from build123d import *

# Parameters (mm, degrees)
SKETCH1_W           = 10.16
SKETCH1_H           = 5.08
BOSS_EXTRUDE1_DEPTH = 63.5
SKETCH2_W           = 2.1082
SKETCH2_H           = 6.073980388
CUT_EXTRUDE1_DEPTH  = 6
SKETCH3_W           = 0.5
SKETCH3_H           = 2.1082
CUT_EXTRUDE2_DEPTH  = 6
SKETCH4_W           = 6.35
SKETCH4_H           = 6.35
BOSS_EXTRUDE2_DEPTH = 60
FILLET3_R           = 4
FILLET4_R           = 0.5
FILLET6_R           = 5
FILLET10_R          = 5


with BuildPart() as part:
    # Sketch1 → Boss-Extrude1 (new body)
    with BuildSketch(Plane(origin=(0, 0, 0), x_dir=(0, 0, -1), z_dir=(1, 0, 0))):
        with Locations((5.08, 2.54)):
            Rectangle(SKETCH1_W, SKETCH1_H)
    extrude(amount=BOSS_EXTRUDE1_DEPTH)

    # Sketch2 → Cut-Extrude1 (cut)
    with BuildSketch(Plane(origin=(0, 5.08, 0), x_dir=(1, 0, 0), z_dir=(0, 1, 0))):
        with Locations((6.1341, 7.123009806)):
            Rectangle(SKETCH2_W, SKETCH2_H)
    extrude(amount=-CUT_EXTRUDE1_DEPTH, mode=Mode.SUBTRACT)

    # Sketch3 → Cut-Extrude2 (cut)
    with BuildSketch(Plane(origin=(0, 5.08, 0), x_dir=(1, 0, 0), z_dir=(0, 1, 0))):
        with Locations((4.83, 5.140119612)):
            Rectangle(SKETCH3_W, SKETCH3_H)
    extrude(amount=-CUT_EXTRUDE2_DEPTH, mode=Mode.SUBTRACT)

    # Sketch4 → Boss-Extrude2 (add)
    with BuildSketch(Plane(origin=(63.5, 0, 0), x_dir=(0, 0, -1), z_dir=(1, 0, 0))):
        with Locations((3.175, 3.175)):
            Rectangle(SKETCH4_W, SKETCH4_H)
    extrude(amount=BOSS_EXTRUDE2_DEPTH)

    # Fillet3
    # the kernel refuses this fillet: 4 mm, written as the material it takes off along each edge
    with BuildSketch(Plane(origin=(7.1882, 15.08, -10.16), x_dir=(0, 0, 1), z_dir=(0, -1, 0)), Plane(origin=(5.08, 15.08, -10.16), x_dir=(-1, 0, 0), z_dir=(0, -1, 0))) as fillet3_piece_1:
        with BuildLine():
            CenterArc((FILLET3_R, -FILLET3_R), FILLET3_R, 90, 90)
            Line((0, -FILLET3_R), (0, 0))
            Line((0, 0), (FILLET3_R, 0))
        make_face()
    extrude(amount=25.08, mode=Mode.SUBTRACT)

    # Fillet4
    # the kernel refuses this fillet: 0.5 mm, written as the material it takes off along each edge
    with BuildSketch(Plane(origin=(5.079853625, -1.440722871, -6.194219612), x_dir=(-0.08056618488507147, 0, -0.9967492612754044), z_dir=(0, 1, 0))) as fillet4_piece_1:
        with BuildLine():
            CenterArc((0.540271076, 0.498701011), FILLET4_R, 180.054119318, 94.076825667)
            Line((0.0402713, 0.498228731), (0.030271304, 0.498219285))
            ThreePointArc((0.030271304, 0.498219285), (0.010168157, 0.249920027), (-0.009967493, 0.000805662))
            Line((-0.009967493, 0.000805662), (-0.000720361, -0.00997402))
            ThreePointArc((-0.000720361, -0.00997402), (0.288144574, -0.020391911), (0.57700951, -0.00997402))
            Line((0.57700951, -0.00997402), (0.576289148, 0))
        make_face()
    extrude(amount=7.961445741, mode=Mode.SUBTRACT)

    # Fillet6
    # the kernel refuses this fillet: 5 mm, written as the material it adds along each edge
    with BuildSketch(Plane(origin=(63.5, 5.08, -6.35), x_dir=(-1, 0, 0), z_dir=(0, 0, 1))) as fillet6_piece_1:
        with BuildLine():
            CenterArc((3.329729719, -5), FILLET6_R, 90, 41.754936598)
            Line((0, -1.27), (0, 0))
            Line((0, 0), (3.329729719, 0))
        make_face()
    extrude(amount=6.35)

    # Fillet10
    # the kernel refuses this fillet: 5 mm, written as the material it adds along each edge
    with BuildSketch(Plane(origin=(63.5, 0, -6.35), x_dir=(1, 0, 0), z_dir=(0, 1, 0))) as fillet10_piece_1:
        with BuildLine():
            CenterArc((4.856325772, 5), FILLET10_R, 193.768528752, 76.231471248)
            Line((0, 3.81), (-0.097126515, 3.7862))
            ThreePointArc((-0.097126515, 3.7862), (-0.1, 1.905), (-0.1, 0))
            Line((-0.1, 0), (0, -0.1))
            Line((0, -0.1), (4.856325772, -0.1))
            Line((4.856325772, -0.1), (4.856325772, 0))
        make_face()
    extrude(amount=5.08)


with BuildPart() as body_2:
    # Mirror1: mirrored copy
    add(part.part.mirror(Plane(origin=(63.5, 0, 0), x_dir=(0, 0, 1), z_dir=(0, 1, 0))))


solid = body_2.part
Could you check a few things on this model? Use its own coordinates, in mm. A direction names the side the tool comes from. Give positions to 0.01 mm unless a question says otherwise; leave off trailing zeros. Order: outer loops, then holes, each group sorted by start corner. A loop starts at its lowest first (then second) coordinate and runs counter-clockwise, first axis right, second up.
1. Suppose I cut it at D-D (x = 115.5). List the corners of the cut face in (y, z) for me, plus the area to 3 significant figures.
2. Suppose I cut it at A-A (y = -3). List the corners of the cut face in (x, z) for me, plus the area to 3 significant figures.
3. Will these pins go through, and if not, where does the flat tip stop? P1, Ø3, axis at x = 98, y = -3.5, coming from the -Z side; P2, Ø3, axis at x = 6.5, y = -3, coming from the -Z side; P3, Ø4, axis at x = 27, z = -2.5, coming from the -Y side.
4. Suppose I cut it at C-C (z = -8.75). List the corners of the cut face in (x, y) for me, plus the area to 3 significant figures.
5. I need wall thicknesses on L1, parallel to Z at x = 72, y = -1.25; L2, parallel to Y at x = 42.5, z = -9.5; L3, parallel to X at y = -1, z = -8. Which ranges of each line are inside material? Lowest first, please.
6. Suppose I cut it at B-B (z = -2.5). List the corners of the cut face in (x, y) for me, plus the area to 3 significant figures.
7. We'd pull the mould along X, two halves only. Please class faces 1 (the flat face through (6, -3, -4.086)), 2 (the flat face through (63, 0, -4)), 3 (the cylindrical face through (65.23, -2.5, -7.45)): pulls with the +X half, pulls with the -X half, needs draft (parallel to the pull), parting line crosses it, or undercut.
8. For faces 4 (the flat face through (7.188, -3, -5)), 5 (the flat face through (4.58, -3, -5)), 6 (the flat face through (0, -3, -5)), which set-ups out of +Z, -Z, +X, -X, +Y, -Y let a thin tool reach every point of the face, with its end or its side?
Solved:
1. outline: (-6.35, -6.35) - (0, -6.35) - (0, 0) - (-6.35, 0) - close
1. area: 40.3 mm2
2. outline: (0, -10.16) - (1.08, -10.16) arc R4 ccw to (5.03, -6.77) arc R0.5 ccw to (4.58, -6.19) - (4.58, -4.09) - (7.19, -4.09) - (7.19, -6.16) arc R4 ccw to (11.19, -10.16) - (63.5, -10.16) arc R5 cw to (68.36, -6.35) - (123.5, -6.35) - (123.5, 0) - (0, 0) - close
2. area: 1,010 mm2
3. P1: stops at z = -6.35
3. P2: stops at z = -8.58
3. P3: stops at y = -5.08
4. outline: (0, -5.08) - (4.13, -5.08) - (4.13, 0) - (0, 0) - close; (8.14, -5.08) - (64.09, -5.08) - (64.09, 0) - (8.14, 0) - close
4. area: 305 mm2
5. L1: z = -6.35 to 0
5. L2: y = -5.08 to 0
5. L3: x = 0 to 4.63, 7.64 to 64.64
6. outline: (0, -5.08) - (60.17, -5.08) arc R5 cw to (63.5, -6.35) - (123.5, -6.35) - (123.5, 0) - (0, 0) - close
6. area: 705 mm2
7. face 1: undercut
7. face 2: needs draft
7. face 3: pulls with the +X half
8. face 4: -Z, +Y, -Y
8. face 5: +Y, -Y
8. face 6: +Z, -Z, -X, +Y, -Y
